```python
from build123d import *

# Parameters (mm, degrees)
SKETCH1_W           = 75
SKETCH1_H           = 95
BOSS_EXTRUDE1_DEPTH = 23
SKETCH3_W           = 55
SKETCH3_H           = 85
CUT_EXTRUDE2_DEPTH  = 19
SKETCH11_W          = 64
SKETCH11_H          = 105
BOSS_EXTRUDE2_DEPTH = 4
SKETCH5_W           = 5.5
SKETCH5_H           = 95
CUT_EXTRUDE4_DEPTH  = 19
SKETCH4_R           = 0.95
SKETCH4_R_2         = 1
CUT_EXTRUDE3_DEPTH  = 10
SKETCH6_R           = 1.25
CUT_EXTRUDE5_DEPTH  = 5
CUT_EXTRUDE6_REACH  = 11
SKETCH7_W           = 50
SKETCH7_H           = 8
SKETCH10_R          = 2.5
CUT_EXTRUDE9_DEPTH  = 2


with BuildPart() as part:
    # Sketch1 → Boss-Extrude1 (new body)
    with BuildSketch(Plane.XY):
        with Locations((37.5, 47.5)):
            Rectangle(SKETCH1_W, SKETCH1_H)
    extrude(amount=BOSS_EXTRUDE1_DEPTH)

    # Sketch3 → Cut-Extrude2 (cut)
    with BuildSketch(Plane(origin=(0, 0, 0), x_dir=(-1, 0, 0), z_dir=(0, 0, -1))):
        with Locations((-37.5, 47.5)):
            Rectangle(SKETCH3_W, SKETCH3_H)
    extrude(amount=-CUT_EXTRUDE2_DEPTH, mode=Mode.SUBTRACT)

    # Sketch11 → Boss-Extrude2 (add)
    with BuildSketch(Plane(origin=(0, 0, 19), x_dir=(-1, 0, 0), z_dir=(0, 0, -1))):
        with Locations((-37.5, 48.5)):
            Rectangle(SKETCH11_W, SKETCH11_H)
    extrude(amount=-BOSS_EXTRUDE2_DEPTH)

    # Sketch5 → Cut-Extrude4 (cut)
    with BuildSketch(Plane.XY.offset(23)):
        with Locations((72.25, 47.5)):
            Rectangle(SKETCH5_W, SKETCH5_H)
        with Locations((2.75, 47.5)):
            Rectangle(SKETCH5_W, SKETCH5_H)
    extrude(amount=-CUT_EXTRUDE4_DEPTH, mode=Mode.SUBTRACT)

    # Sketch4 → Cut-Extrude3 (cut)
    with BuildSketch(Plane(origin=(0, 0, 23), x_dir=(-1, 0, 0), z_dir=(0, 0, -1))):
        with Locations((-9, 97.31)):
            Circle(SKETCH4_R)
        with Locations((-67, 97.31)):
            Circle(SKETCH4_R)
        with Locations((-67, 42.51)):
            Circle(SKETCH4_R)
        with Locations((-67, 13.01)):
            Circle(SKETCH4_R)
        with Locations((-9, 13.01)):
            Circle(SKETCH4_R)
        with Locations((-14.5, 15)):
            Circle(SKETCH4_R_2)
        with Locations((-54.5, 15)):
            Circle(SKETCH4_R_2)
    extrude(amount=CUT_EXTRUDE3_DEPTH, mode=Mode.SUBTRACT)

    # Sketch6 → Cut-Extrude5 (cut, through all)
    with BuildSketch(Plane.XY.offset(4)):
        with Locations((72, 10)):
            Circle(SKETCH6_R)
        with Locations((3, 10)):
            Circle(SKETCH6_R)
        with Locations((72, 35)):
            Circle(SKETCH6_R)
        with Locations((3, 35)):
            Circle(SKETCH6_R)
        with Locations((72, 60)):
            Circle(SKETCH6_R)
        with Locations((3, 60)):
            Circle(SKETCH6_R)
        with Locations((72, 85)):
            Circle(SKETCH6_R)
        with Locations((3, 85)):
            Circle(SKETCH6_R)
    extrude(amount=-CUT_EXTRUDE5_DEPTH, mode=Mode.SUBTRACT)

    # Sketch7 → Cut-Extrude6 (cut, up to next)
    with BuildSketch(Plane(origin=(0, 5, 0), x_dir=(1, 0, 0), z_dir=(0, 1, 0)), mode=Mode.PRIVATE) as cut_extrude6_sk1:
        with Locations((35, -15)):
            Rectangle(SKETCH7_W, SKETCH7_H)
    cut_extrude6_tool1 = extrude(cut_extrude6_sk1.sketch, amount=-CUT_EXTRUDE6_REACH, mode=Mode.PRIVATE) & part.part
    add(cut_extrude6_tool1.solids().sort_by_distance((35, 5, 15))[0], mode=Mode.SUBTRACT)

    # Sketch10 → Cut-Extrude9 (cut)
    with BuildSketch(Plane.XY.offset(4)):
        with Locations((72, 10)):
            Circle(SKETCH10_R)
        with Locations((72, 35)):
            Circle(SKETCH10_R)
        with Locations((72, 60)):
            Circle(SKETCH10_R)
        with Locations((72, 85)):
            Circle(SKETCH10_R)
        with Locations((3, 10)):
            Circle(SKETCH10_R)
        with Locations((3, 35)):
            Circle(SKETCH10_R)
        with Locations((3, 60)):
            Circle(SKETCH10_R)
        with Locations((3, 85)):
            Circle(SKETCH10_R)
    extrude(amount=-CUT_EXTRUDE9_DEPTH, mode=Mode.SUBTRACT)


solid = part.part
```
Could you check a few things on this model? Use its own coordinates, in mm. A direction names the side the tool comes from. Round coordinates to 2 decimals unless told otherwise and drop trailing zeros. Loops run counter-clockwise (first coordinate to the right, second up) from the corner with the lowest first, then second, coordinate; pieces in that order, holes last. Notation, with made-up numbers: (-32.5, -16.75) - (-12.5, -16.75) arc R30 cw to (-12.5, 18.25) - close; hole circle Ø10 at (40.5, 76.5). An arc over 180 degrees is marked (long way). Use CSV: the item, a comma, the result in double quotes.
Item 1: Will these pins go through, and if not, where does the flat tip stop? pin 1 (1.6 mm diameter, centred on x = 14.5, y = 15, fed in from -Z) (3 decimals); pin 2 (2.5 mm diameter, centred on x = 3, y = 85.5, fed in from +Z); pin 3 (1.5 mm diameter, centred on x = 41, z = 3, fed in from -Y); pin 4 (1.5 mm diameter, centred on x = 37.5, z = 17.5, fed in from +Y).
Here are the results:
pin 1,"passes through"
pin 2,"stops at z = 2"
pin 3,"stops at y = 0"
pin 4,"stops at y = 95"
Item 2: I need wall thicknesses on L1, parallel to Y at x = 3, z = 3.25; L2, parallel to Y at x = 62, z = 10.75; L3, parallel to Y at x = 9, z = 22.25. Which ranges of each line are inside material? Lowest first, please. Write a range as [from, to].
Here are the results:
L1,"y = [0, 7.5], [12.5, 32.5], [37.5, 57.5], [62.5, 82.5], [87.5, 95]"
L2,"y = [0, 5], [90, 95]"
L3,"y = [-4, 12.06], [13.96, 96.36], [98.26, 101]"
Item 3: If we section it at B-B on y = 50.5: List the corners of the cut face in (x, z) for me, then the cut area to 3 significant figures.
Here are the results:
outline,"(0, 0) - (10, 0) - (10, 19) - (65, 19) - (65, 0) - (75, 0) - (75, 4) - (69.5, 4) - (69.5, 23) - (5.5, 23) - (5.5, 4) - (0, 4) - close"
area,"471 mm²"
Item 4: If we section it at C-C on x = 3: Count the separate pieces of the cut face and the enclosed holes in it, then the cut area to 3 significant figures.
Here are the results:
separate pieces,"5"
enclosed holes,"0"
area,"320 mm²"
Item 5: If we section it at A-A on x = 39: List the corners of the cut face in (y, z) for me.
Here are the results:
outline,"(-4, 19) - (90, 19) - (90, 0) - (95, 0) - (95, 19) - (101, 19) - (101, 23) - (-4, 23) - close; (0, 0) - (5, 0) - (5, 11) - (0, 11) - close"
Item 6: If we mould it in two halves opening along X, with no side actions, what happens to faces 1 (the flat face through (0, 47, 2)), 2 (the flat face through (38, 49, 23)), 3 (the cylindrical face through (71.67, 87.48, 3.01)), 4 (the flat face through (69.5, 48, 13))? For each: pulls with the +X half, pulls with the -X half, needs draft (parallel to the pull), parting line crosses it, or undercut.
Here are the results:
face 1,"pulls with the -X half"
face 2,"needs draft"
face 3,"undercut"
face 4,"pulls with the +X half"
Item 7: For faces 5 (the flat face through (5.5, 48, 13)), 6 (the flat face through (4, 61, 2)), 7 (the flat face through (38, 90, 9)), 8 (the flat face through (38, 98, 19)), which set-ups out of +Z, -Z, +X, -X, +Y, -Y let a thin tool reach every point of the face, with its end or its side?
Here are the results:
face 5,"+Z, -X, +Y, -Y"
face 6,"+Z"
face 7,"-Z"
face 8,"-Z, +X, -X, +Y"
